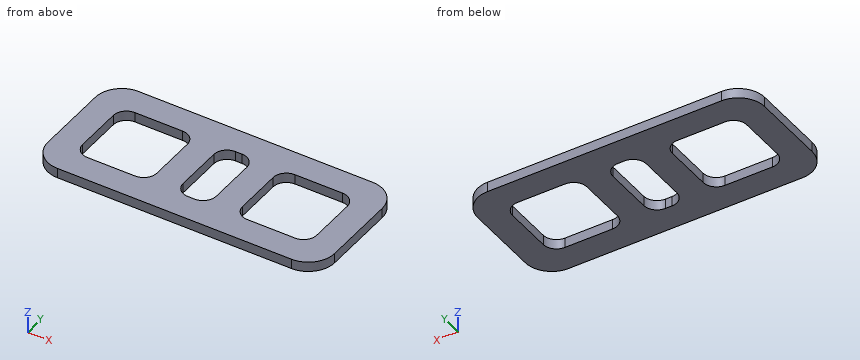
Autodesk Inventor part; units mm, degrees
ref_plane "YZ Plane" through (0, 0, 0) normal (1, 0, 0) x (0, 1, 0)
ref_plane "XZ Plane" through (0, 0, 0) normal (0, 1, 0) x (-1, 0, 0)
ref_plane "XY Plane" through (0, 0, 0) normal (0, 0, 1) x (1, 0, 0)
sketch "Sketch2" plane through (0, 0, 0) normal (0, 0, 1) x (1, 0, 0)
  line L0 (0, 0) -> (552.641777, 0)
  line L1 (552.641777, 0) -> (552.641777, 244.475)
  line L2 (552.641777, 244.475) -> (0, 244.475)
  line L3 (0, 244.475) -> (0, 0)
  dimension "d6" = 244.475
extrude "Extrusion1" add sketch "Sketch2" along normal blind 19.05
sketch "Sketch3" plane through (0, 0, 19.05) normal (0, 0, 1) x (1, 0, 0)
  line L0 (0, 0) -> (552.641777, 0)
  line L1 (552.641777, 0) -> (552.641777, 244.475)
  line L2 (552.641777, 244.475) -> (0, 244.475)
  line L3 (0, 244.475) -> (0, 0)
  arc A0 (50.896482, 244.475) -> (0, 193.636302) centre (50.799985, 193.675092) ccw
  dimension "d9" = 50.8
sketch "Sketch3 outline for Extrusion2" plane through (0, 0, 19.05) normal (0, 0, 1) x (1, 0, 0)
  arc A0 (50.896482, 244.475) -> (0, 193.636302) centre (50.799985, 193.675092) ccw
  line L0 (0, 244.475) -> (0, 193.636302)
  line L1 (50.896482, 244.475) -> (0, 244.475)
extrude "Extrusion2" cut sketch "Sketch3 outline for Extrusion2" against normal blind 19.05
sketch "Sketch4" plane through (0, 0, 19.05) normal (0, 0, 1) x (1, 0, 0)
  line L0 (0, 193.713882) -> (0, 0)
  line L1 (0, 0) -> (552.641777, 0)
  line L2 (552.641777, 0) -> (552.641777, 244.475)
  line L3 (552.641777, 244.475) -> (50.703488, 244.475)
  arc A0 (552.641777, 193.713882) -> (500.210663, 244.475) centre (501.841779, 193.701193) ccw
  arc A1 (501.841779, 0) -> (552.641777, 50.788429) centre (501.841778, 50.8) ccw
  arc A2 (0, 50.788429) -> (50.703488, 0) centre (50.799999, 50.799908) ccw
  dimension "d15" = 50.8
  dimension "d16" = 50.8
  dimension "d17" = 50.8
extrude "Extrusion3" cut sketch "Sketch4" against normal blind 19.05 contours A2 L1 L0
sketch "Sketch5" plane through (0, 0, 19.05) normal (0, 0, 1) x (1, 0, 0)
  line L0 (552.641777, 0) -> (552.641777, 244.475)
  line L1 (552.641777, 244.475) -> (50.703488, 244.475)
  arc A0 (552.641777, 193.713882) -> (501.92669, 244.475) centre (501.841792, 193.675071) ccw
  point P0 (0, 0)
  dimension "d20" = 50.8
extrude "Extrusion4" cut sketch "Sketch5" against normal blind 19.05
sketch "Sketch6" plane through (0, 0, 19.05) normal (0, 0, 1) x (1, 0, 0)
  line L0 (50.703488, 0) -> (552.641777, 0)
  line L1 (552.641777, 0) -> (552.641777, 193.713882)
  arc A0 (501.92669, 0) -> (552.641777, 50.799908) centre (501.841777, 50.799929) ccw
  point P0 (0, 0)
  dimension "d23" = 50.8
extrude "Extrusion5" cut sketch "Sketch6" against normal blind 19.05
sketch "Sketch7" plane through (0, 0, 19.05) normal (0, 0, 1) x (1, 0, 0)
  arc A0 (552.641777, 193.713882) -> (501.92669, 244.475) centre (501.841792, 193.675071) ccw
  arc A1 (50.703488, 244.475) -> (0, 193.713882) centre (50.799985, 193.675092) ccw
  line L0 (50.799985, 193.675092) -> (193.674985, 193.675092)
  line L1 (193.674985, 193.675092) -> (193.674985, 50.799908)
  line L2 (193.674985, 50.799908) -> (50.799985, 50.799908)
  line L3 (50.799985, 50.799908) -> (50.799985, 193.675092)
  line L4 (501.841792, 193.675071) -> (358.966792, 193.675071)
  line L5 (358.966792, 193.675071) -> (358.966792, 50.799908)
  line L6 (358.966792, 50.799908) -> (501.841792, 50.799908)
  line L7 (501.841792, 50.799908) -> (501.841792, 193.675071)
  point P0 (0, 0)
  dimension "d26" = 142.875
  dimension "d27" = 142.875
extrude "Extrusion6" cut sketch "Sketch7" against normal blind 19.05 contours L0 L1 L2 L3
sketch "Sketch8" plane through (0, 0, 19.05) normal (0, 0, 1) x (1, 0, 0)
  arc A0 (552.641777, 193.713882) -> (501.92669, 244.475) centre (501.841792, 193.675071) ccw
  line L0 (501.841792, 193.675071) -> (358.966792, 193.675071)
  line L1 (358.966792, 193.675071) -> (358.966792, 50.799908)
  line L2 (358.966792, 50.799908) -> (501.841792, 50.799908)
  line L3 (501.841792, 50.799908) -> (501.841792, 193.675071)
  point P0 (0, 0)
  dimension "d30" = 142.875
extrude "Extrusion7" cut sketch "Sketch8" against normal blind 19.05
sketch "Sketch9" plane through (0, 0, 19.05) normal (0, 0, 1) x (1, 0, 0)
  line L0 (244.474985, 193.675092) -> (308.166792, 193.675092)
  line L1 (308.166792, 193.675092) -> (308.166792, 50.799908)
  line L2 (308.166792, 50.799908) -> (244.474985, 50.799908)
  line L3 (244.474985, 50.799908) -> (244.474985, 193.675092)
  point P0 (193.674985, 193.675092)
  point P1 (0, 0)
  dimension "d33" = 50.8
extrude "Extrusion8" cut sketch "Sketch9" against normal blind 19.05
fillet "Fillet1" radius 25.4 1 edges at (50.8, 193.6751, 9.525)
fillet "Fillet2" radius 25.4 1 edges at (193.675, 193.6751, 9.525)
fillet "Fillet3" radius 25.4 1 edges at (308.1668, 193.6751, 9.525)
fillet "Fillet4" radius 25.4 1 edges at (501.8418, 193.6751, 9.525)
fillet "Fillet5" radius 25.4 1 edges at (501.8418, 50.7999, 9.525)
fillet "Fillet6" radius 25.4 1 edges at (358.9668, 193.6751, 9.525)
fillet "Fillet7" radius 25.4 1 edges at (358.9668, 50.7999, 9.525)
fillet "Fillet8" radius 25.4 1 edges at (244.475, 50.7999, 9.525)
fillet "Fillet9" radius 25.4 1 edges at (244.475, 193.6751, 9.525)
fillet "Fillet10" radius 25.4 1 edges at (193.675, 50.7999, 9.525)
fillet "Fillet11" radius 25.4 1 edges at (308.1668, 50.7999, 9.525)
fillet "Fillet12" radius 25.4 1 edges at (50.8, 50.7999, 9.525)
properties part number "ROV-Side Panel" material "Acetal Resin, Black"
Design review of the part built by this model. Coordinates are the model's own, in mm. Give positions to 0.01 mm unless a question says otherwise; leave off trailing zeros. Order: outer loops, then holes, each group sorted by start corner. A loop starts at its lowest first (then second) coordinate and runs counter-clockwise, first axis right, second up. Notation, with made-up numbers: (82, 72) -> (131, 72) arc R11 ccw to (131, 86) -> close; hole circle Ø7 at (12.5, 58.5). An arc over 180 degrees is marked (long way). Write item = value, one per line. Start each with the question number.
(1) To check wall thickness, follow line 1 along X through (y, z) = (107, 15.75); line 2 along Y through (x, z) = (403, 14.5) (3 decimals); line 3 along X through (y, z) = (69, 6). State the ranges of each line that lie inside material, in increasing order.
(2) We need section B-B on z = 7.25. State how many separate pieces and enclosed holes the cut face has, plus the area to 3 significant figures.
(3) We need section A-A on x = 459. Write out the cut boundary in (y, z) (3 decimals), plus the area to 3 significant figures.
Numbers:
q1.line_1 = 0 to 50.8, 193.67 to 244.47, 308.17 to 358.97, 501.84 to 552.64
q1.line_2 = 0 to 50.8, 193.675 to 244.475
q1.line_3 = 0 to 51.84, 192.63 to 245.52, 307.12 to 360.01, 500.8 to 552.64
q2.separate_pieces = 1
q2.enclosed_holes = 3
q2.area = 84,600 mm^2
q3.outline = (0, 0) -> (50.8, 0) -> (50.8, 19.05) -> (0, 19.05) -> close; (193.675, 0) -> (244.475, 0) -> (244.475, 19.05) -> (193.675, 19.05) -> close
q3.area = 1,940 mm^2
